```python
from build123d import *

# Parameters (mm, degrees)
BOSS_EXTRUDE1_DEPTH  = 15
CUT_EXTRUDE1_DEPTH   = 43.992404265
SKETCH3_R            = 5
CUT_EXTRUDE2_DEPTH   = 36.004455062
SKETCH5_W            = 10.737519515
SKETCH5_H            = 30
SKETCH5_W_2          = 6.95
CUT_EXTRUDE3_DEPTH   = 36.004455062
SKETCH7_R            = 2.5
CUT_EXTRUDE4_DEPTH   = 24.248431868
BOSS_EXTRUDE4_DEPTH  = 15
SKETCH9_R            = 2.5
CUT_EXTRUDE5_DEPTH   = 15
FILLET1_R            = 5
FILLET1_OF_MIRROR1_R = 5


with BuildPart() as part:
    # Sketch1 → Boss-Extrude1 (new, symmetric)
    with BuildSketch(Plane(origin=(0, 0, 0), x_dir=(1, 0, 0), z_dir=(0, 1, 0))):
        Polygon((-9.48841315, -9.301961234), (-0.940151386, -8.006660352), (17.861436312, 17.510450435), (15.605946265, 22.576364023), (9.067678571, 25.086169843), (2.607936691, 22.210107458), align=None)
    extrude(amount=BOSS_EXTRUDE1_DEPTH, both=True)

    # Sketch2 → Cut-Extrude1 (cut, through all)
    with BuildSketch(Plane.XZ.offset(15)):
        Polygon((-9.48841315, 9.301961234), (2.607936691, -22.210107458), (9.067678571, -25.086169843), (15.605946265, -22.576364023), (17.861436312, -17.510450435), (-0.940151386, 8.006660352), align=None)
        Polygon((-8.713652873, 8.678855764), (3.000506472, -21.837572646), (9.081845433, -24.545159197), (15.233411453, -22.183794243), (17.286339277, -17.572842857), (-1.219829574, 7.543331818), align=None, mode=Mode.SUBTRACT)
    extrude(amount=-CUT_EXTRUDE1_DEPTH, mode=Mode.SUBTRACT)

    # Sketch3 → Cut-Extrude2 (cut, through all)
    with BuildSketch(Plane(origin=(-4.690935448, 0, -1.800681409), x_dir=(-0.3583679495453122, 0, 0.9335804264971972), z_dir=(-0.9335804264971972, 0, -0.3583679495453122))):
        with Locations((-3.224896221, 0)):
            Circle(SKETCH3_R)
    extrude(amount=-CUT_EXTRUDE2_DEPTH, mode=Mode.SUBTRACT)

    # Sketch5 → Cut-Extrude3 (cut, through all)
    with BuildSketch(Plane(origin=(-4.690935448, 0, -1.800681409), x_dir=(-0.35836794954531215, 0, 0.9335804264971973), z_dir=(-0.9335804264971973, 0, -0.35836794954531215))):
        with Locations((-16.093655978, 0)):
            Rectangle(SKETCH5_W, SKETCH5_H)
        with Locations((7.750103779, 0)):
            Rectangle(SKETCH5_W_2, SKETCH5_H)
    extrude(amount=-CUT_EXTRUDE3_DEPTH, mode=Mode.SUBTRACT)


with BuildPart() as cut_extrude3_kept_piece:
    # of the separate pieces the step leaves, the one the design keeps (cut_extrude3_pieces_kept)
    add(part.part.solids().sort_by_distance((-6.222995624, -15, 2.1904718))[0])

    # Sketch7 → Cut-Extrude4 (cut, through all)
    with BuildSketch(Plane(origin=(-4.690935448, 0, -1.800681409), x_dir=(-0.35836794954531215, 0, 0.9335804264971973), z_dir=(-0.9335804264971973, 0, -0.35836794954531215))):
        with Locations((-3.224896221, 10)):
            Circle(SKETCH7_R)
        with Locations((-3.224896221, -10)):
            Circle(SKETCH7_R)
    extrude(amount=-CUT_EXTRUDE4_DEPTH, mode=Mode.SUBTRACT)

    # Sketch8 → Boss-Extrude4 (add)
    with BuildSketch(Plane(origin=(0, 15, 0), x_dir=(1, 0, 0), z_dir=(0, 1, 0))):
        Polygon((-2.639316128, 7.145332465), (-6.222995624, -2.1904718), (0.751589516, -4.867764195), (4.335269011, 4.46804007), align=None)
    boss_extrude4 = extrude(amount=BOSS_EXTRUDE4_DEPTH)

    # Sketch9 → Cut-Extrude5 (cut)
    with BuildSketch(Plane(origin=(2.283649691, 0, 0.876610985), x_dir=(0.3583679495453119, 0, -0.9335804264971973), z_dir=(0.9335804264971973, 0, 0.3583679495453119))):
        with Locations((0.724896221, 25)):
            Circle(SKETCH9_R)
    cut_extrude5 = extrude(amount=-CUT_EXTRUDE5_DEPTH, mode=Mode.SUBTRACT)

    # Fillet1
    fillet1_edges = [cut_extrude3_kept_piece.edges().sort_by_distance(p)[0] for p in [
        (-2.735703054, 30, 3.529117997),
        (0.847976442, 30, -5.806686268),
    ]]
    fillet(fillet1_edges, radius=FILLET1_R - 0.0001)  # a hair under: the kernel refuses the full size

    # Mirror1: Boss-Extrude4, Cut-Extrude5 across plane
    add(boss_extrude4.mirror(Plane.ZX))
    add(cut_extrude5.mirror(Plane.ZX), mode=Mode.SUBTRACT)

    # Fillet1 of Mirror1
    fillet1_of_mirror1_edges = [cut_extrude3_kept_piece.edges().sort_by_distance(p)[0] for p in [
        (-2.735703054, -30, 3.529117997),
        (0.847976442, -30, -5.806686268),
    ]]
    fillet(fillet1_of_mirror1_edges, radius=FILLET1_OF_MIRROR1_R - 0.0001)  # a hair under: the kernel refuses the full size


solid = cut_extrude3_kept_piece.part
```
Build history of the part. All positions in model axes, mm. A direction names the side the tool comes from. Coordinates: 2 decimals unless noted, no trailing zeros. Order: outer loops, then holes, each group sorted by start corner. A loop starts at its lowest first (then second) coordinate and runs counter-clockwise, first axis right, second up. Notation, with made-up numbers: (71.5, 80) -> (86.5, 80) arc R22 ccw to (86.5, 102) -> close; hole circle Ø4 at (-23.75, 32.5). An arc over 180 degrees is marked (long way). Answer in a Markdown table with one row per item. Add a question column.
Q1. Wall check: line 1 along Y through (x, z) = (0.75, 1.5); line 2 along Y through (x, z) = (-4, -0.25); line 3 along Z through (x, y) = (1.75, -12). Give the ranges that are in metal, low to high. Write a range as [from, to].
Q2. Band-saw the part on A-A, the plane y = -2. List the corners of the cut face in (x, z).
Q3. Band-saw the part on B-B, the plane z = -1.25. Give the number of separate pieces and of enclosed holes in the cut face, then the cut area to 3 significant figures.
Q4. Mould opens along X. For faces 1 (the face through (-2.148, 28.574, 2.144)), 2 (the face through (4.491, -0.21, -9.764)), 3 (the face through (1.91, 8.479, -4.846)) say: +X half, -X half, draft (parallel to the pull), parting line (faces both ways), or undercut.
Q5. Which spindle directions (+Z, -Z, +X, -X, +Y, -Y) get a long thin tool onto all of the face, cutting with end or side? Do faces 4 (the face through (0.897, -19.93, -5.788)), 5 (the face through (0.897, 19.93, -5.788)), 6 (the face through (2.518, 20.728, 0.265)), 7 (the face through (2.518, -20.728, 0.265)). Say none if no direction does.
Q6. Band-saw the part on C-C, the plane y = 21. List the corners of the cut face in (x, z), then the cut area to 3 significant figures.
Q7. Drop flat-ended pins along their axis: pin 1 (4 mm diameter, centred on x = 5.5, z = -4.5, fed in from +Y); pin 2 (4 mm diameter, centred on y = -0.5, z = 1.5, fed in from -X); pin 3 (2 mm diameter, centred on x = -4, z = -4.5, fed in from +Y). Give the stop position or say it passes through.
Answers follow:
| question | item | result |
|---|---|---|
| 1 | line 1 | [-29.64, -26.67], [-23.33, -2.45], [2.45, 23.33], [26.67, 29.64] |
| 1 | line 2 | [-29.61, -26.6], [-23.4, -2.33], [2.33, 23.4], [26.6, 29.61] |
| 1 | line 3 | [-10.82, -4.39], [-1.18, 3.51] |
| 2 | outline | (-6.22, 2.19) -> (-5.18, -0.53) -> (2.55, 2.43) -> (0.75, 4.87) -> close; (-1.89, -9.09) -> (-0.85, -11.81) -> (9.98, -7.66) -> (8.19, -5.22) -> close |
| 3 | separate pieces | 4 |
| 3 | enclosed holes | 0 |
| 3 | area | 328 mm^2 |
| 4 | face 1 | -X half |
| 4 | face 2 | +X half |
| 4 | face 3 | undercut |
| 5 | face 4 | -Z, +X, -Y |
| 5 | face 5 | -Z, +X, +Y |
| 5 | face 6 | +Z, +X, +Y |
| 5 | face 7 | +Z, +X, -Y |
| 6 | outline | (-6.22, 2.19) -> (-2.64, -7.15) -> (4.34, -4.47) -> (0.75, 4.87) -> close |
| 6 | area | 74.7 mm^2 |
| 7 | pin 1 | y = 28.29 |
| 7 | pin 2 | x = -6.22 |
| 7 | pin 3 | y = 29.88 |
